from build123d import *

# Parameters (mm, degrees)
SKETCH1_W           = 193.9764
SKETCH1_H           = 32.5
BOSS_EXTRUDE1_DEPTH = 6.35
SKETCH2_R           = 2.75
CUT_EXTRUDE1_DEPTH  = 197.782662491
BOSS_EXTRUDE2_DEPTH = 5.715
SKETCH4_R           = 2.75
CUT_EXTRUDE2_DEPTH  = 208.356239103


with BuildPart() as part:
    # Sketch1 → Boss-Extrude1 (new body)
    with BuildSketch(Plane.XY):
        with Locations((96.9882, 16.25)):
            Rectangle(SKETCH1_W, SKETCH1_H)
    extrude(amount=BOSS_EXTRUDE1_DEPTH)

    # Sketch2 → Cut-Extrude1 (cut, through all)
    with BuildSketch(Plane.XY.offset(6.35)):
        with Locations((6, 25)):
            Circle(SKETCH2_R)
        with Locations((6, 7)):
            Circle(SKETCH2_R)
    extrude(amount=-CUT_EXTRUDE1_DEPTH, mode=Mode.SUBTRACT)

    # Sketch3 → Boss-Extrude2 (add)
    with BuildSketch(Plane(origin=(193.9764, 0, 0), x_dir=(0, 0, -1), z_dir=(1, 0, 0))):
        Polygon((-28.575, 39.500902), (-28.575, 22.594), (22.225, 22.594), (22.225, 39.500902), (-3.175, 39.500902), align=None)
        Polygon((22.225, 22.594), (-28.575, 22.594), (-6.35, 0), (0, 0), align=None)
        Polygon((-28.575, 47.994), (-28.575, 39.500902), (-3.175, 39.500902), (22.225, 39.500902), (22.225, 47.994), align=None)
    extrude(amount=BOSS_EXTRUDE2_DEPTH)

    # Sketch4 → Cut-Extrude2 (cut, through all)
    with BuildSketch(Plane(origin=(199.6914, 0, 0), x_dir=(0, 0, -1), z_dir=(1, 0, 0))):
        with Locations((-19.05, 35.294)):
            Circle(SKETCH4_R)
        with Locations((12.7, 35.294)):
            Circle(SKETCH4_R)
    extrude(amount=-CUT_EXTRUDE2_DEPTH, mode=Mode.SUBTRACT)


solid = part.part
For this review, take the finished solid that the model builds, in its own axes (mm). A direction names the side the tool comes from. Round coordinates to 2 decimals unless told otherwise and drop trailing zeros. Loops run counter-clockwise (first coordinate to the right, second up) from the corner with the lowest first, then second, coordinate; pieces in that order, holes last. Notation, with made-up numbers: (-27.75, 14.5) - (-7.75, 14.5) arc R15 cw to (-7.75, 19.5) - close; hole circle Ø2 at (48.5, -39.5). An arc over 180 degrees is marked (long way). Put each result on its own line as item: value. Start each with the question number.
1. Consider section D-D on z = -12.7. State the section outline as (x, y) points.
2. For faces 5 (the flat face through (96, 16, 0)), 6 (the flat face through (96, 16, 6.35)), 7 (the cylindrical face through (8.54, 5.95, 3.22)), list the 3-axis set-ups (+Z, -Z, +X, -X, +Y, -Y) from which the entire face can be reached by the end or side of a thin tool; tool diameter is ignored.
3. Consider section A-A on y = 25. State the section outline as (x, z) points (3 decimals).
4. Mouldability with a two-part tool opening along Y and no side actions: class faces 1 (the flat face through (98, 0, 3)), 2 (the flat face through (96, 32.5, 3)), 3 (the flat face through (199.691, 30, 4)), 4 (the cylindrical face through (196.9, 32.6, 19.6)) as +Y half, -Y half, draft (parallel to the pull), parting line (faces both ways), or undercut.
5. Consider section B-B on x = 6. State the section outline as (y, z) points, plus the area to 3 significant figures.
6. Consider section C-C on z = 3. State the section outline as (x, y) points.
7. For probe 1 along Y at (x, z) = (6, 5); probe 2 along X at (y, z) = (10.5, -7); probe 3 along Z at (x, y) = (170.5, 9.5), list the stretches that pass through material, from the lowest coordinate up. Write a range as [from, to].
8. Insertion check: P1, Ø8, axis at x = 143.5, z = -1, coming from the +Y side; P2, Ø16, axis at x = 69, y = 17, coming from the +Z side; P3, Ø2, axis at x = 155.5, y = 33, coming from the -Z side. Each pin has a flat end and moves straight along its axis. Give the tip position at first contact, or say it passes through.
Result sheet:
1. outline: (193.98, 12.91) - (199.69, 12.91) - (199.69, 32.54) - (193.98, 32.54) - close; (193.98, 38.04) - (199.69, 38.04) - (199.69, 47.99) - (193.98, 47.99) - close
2. face 5: -Z, -X, +Y, -Y
2. face 6: +Z, -X, +Y, -Y
2. face 7: +Z, -Z
3. outline: (0, 0) - (3.25, 0) - (3.25, 6.35) - (0, 6.35) - close; (8.75, 0) - (193.976, 0) - (193.976, -22.225) - (199.691, -22.225) - (199.691, 28.575) - (193.976, 28.575) - (193.976, 6.35) - (8.75, 6.35) - close
4. face 1: -Y half
4. face 2: +Y half
4. face 3: draft
4. face 4: undercut
5. outline: (0, 0) - (4.25, 0) - (4.25, 6.35) - (0, 6.35) - close; (9.75, 0) - (22.25, 0) - (22.25, 6.35) - (9.75, 6.35) - close; (27.75, 0) - (32.5, 0) - (32.5, 6.35) - (27.75, 6.35) - close
5. area: 137 mm^2
6. outline: (0, 0) - (199.69, 0) - (199.69, 47.99) - (193.98, 47.99) - (193.98, 32.5) - (0, 32.5) - close; hole circle Ø5.5 at (6, 7); hole circle Ø5.5 at (6, 25)
7. probe 1: [0, 4.25], [9.75, 22.25], [27.75, 32.5]
7. probe 2: [193.98, 199.69]
7. probe 3: [0, 6.35]
8. P1: y = 32.5
8. P2: z = 6.35
8. P3: z = 0
